Part model, mm, in its own coordinate system. A direction names the side the tool comes from. Coordinates: 2 decimals unless noted, no trailing zeros. Loops run counter-clockwise (first coordinate to the right, second up) from the corner with the lowest first, then second, coordinate; pieces in that order, holes last. Notation, with made-up numbers: (45, -21.5) - (50, -21.5) arc R22 ccw to (50, -4.5) - close; hole circle Ø8 at (56.5, 19). An arc over 180 degrees is marked (long way). Use a Markdown table: item, result. Add a question column.
1. Band-saw the part on A-A, the plane x = 0. Give the cut face in (y, z) (1 decimal), plus the area to 3 significant figures.
2. Drop flat-ended pins along their axis: pin 1 (2.5 mm diameter, centred on y = 15, z = -7.5, fed in from +X); pin 2 (3 mm diameter, centred on x = 9.5, y = 15, fed in from +Z); pin 3 (1.6 mm diameter, centred on y = 16, z = -7, fed in from -X). Give the stop position or say it passes through.
3. Band-saw the part on C-C, the plane y = 32.5. Give the cut face in (x, z) (1 decimal).
4. Wall check: probe 1 along Y at (x, z) = (-9.5, -7.1) (3 decimals); probe 2 along X at (y, z) = (32, 0); probe 3 along X at (y, z) = (6.3, -7.15). Give the ranges that are in metal, low to high. Write a range as [from, to].
5. 3-axis set-ups, long thin cutter, end or side, ignore diameter. For faces 4 (the flat face through (-10, 28.575, -7)), 5 (the flat face through (-8, 19, -5.397)), 6 (the flat face through (0, 9.525, -3)): which of +Z, -Z, +X, -X, +Y, -Y reach the whole face in a straight line?
6. Band-saw the part on D-D, the plane z = 4.5. Give the cut face in (x, y) (3 decimals), plus the area to 3 significant figures.
7. Pull direction Y, two halves, no side cores. Call faces 1 (the cylindrical face through (-11.976, 0.764, -7.007)), 2 (the cylindrical face through (11.516, 30.254, -7.007)), 3 (the flat face through (8, 19, -5.397)): pulls with the +Y half, pulls with the -Y half, needs draft (parallel to the pull), parting line crosses it, or undercut.
8. Band-saw the part on B-B, the plane z = 0. Give the cut face in (x, y) (1 decimal).
from build123d import *

# Parameters (mm, degrees)
SKETCH1_R           = 2.2225
BOSS_EXTRUDE1_DEPTH = 38.1
SKETCH3_W           = 12.7
SKETCH3_H           = 19.05
CUT_EXTRUDE2_DEPTH  = 43.521276806
SKETCH8_W           = 3.81
SKETCH8_H           = 19.05
CUT_EXTRUDE4_DEPTH  = 42.586422571
FILLET1_R           = 2.54
FILLET2_R           = 2.54
FILLET3_R           = 2.54
FILLET4_R           = 2.54
FILLET5_R           = 2.54
FILLET6_R           = 2.54
FILLET7_R           = 2.54
FILLET8_R           = 2.54
SKETCH9_R           = 2.54
CUT_EXTRUDE5_DEPTH  = 43.521276806


with BuildPart() as part:
    # Sketch1 → Boss-Extrude1 (new body)
    with BuildSketch(Plane(origin=(0, 0, 0), x_dir=(1, 0, 0), z_dir=(0, 1, 0))):
        with BuildLine():
            Line((-12.7, 8.572431324), (12.7, 8.572431324))
            Line((12.7, 8.572431324), (12.7, 5.397431324))
            Line((12.7, 5.397431324), (6.600302959, 5.397431324))
            ThreePointArc((6.600302959, 5.397431324), (4.87882252, 4.432224955), (4.804297319, 2.460027138))
            ThreePointArc((4.804297319, 2.460027138), (0, -5.3975), (-4.804297319, 2.460027138))
            ThreePointArc((-4.804297319, 2.460027138), (-4.87882252, 4.432224955), (-6.600302959, 5.397431324))
            Line((-6.600302959, 5.397431324), (-12.7, 5.397431324))
            Line((-12.7, 5.397431324), (-12.7, 8.572431324))
        make_face()
        with Locations(Location((0, 0, 0), (0, 0, 90))):
            Circle(SKETCH1_R, mode=Mode.SUBTRACT)
    extrude(amount=BOSS_EXTRUDE1_DEPTH)

    # Sketch3 → Cut-Extrude2 (cut, through all)
    with BuildSketch(Plane(origin=(0, 0, -8.572431324), x_dir=(-1, 0, 0), z_dir=(0, 0, -1))):
        with Locations((0, 19.05)):
            Rectangle(SKETCH3_W, SKETCH3_H)
    extrude(amount=-CUT_EXTRUDE2_DEPTH, mode=Mode.SUBTRACT)

    # Sketch8 → Cut-Extrude4 (cut, through all)
    with BuildSketch(Plane.XY.offset(-5.397431324)):
        with Locations((-10.795, 19.05)):
            Rectangle(SKETCH8_W, SKETCH8_H)
        with Locations((10.795, 19.05)):
            Rectangle(SKETCH8_W, SKETCH8_H)
    extrude(amount=-CUT_EXTRUDE4_DEPTH, mode=Mode.SUBTRACT)

    # Fillet1
    fillet1_edges = [part.edges().sort_by_distance(p)[0] for p in [
        (12.7, 38.1, -6.984931324),
    ]]
    fillet(fillet1_edges, radius=FILLET1_R)

    # Fillet2
    fillet2_edges = [part.edges().sort_by_distance(p)[0] for p in [
        (-12.7, 38.1, -6.984931324),
    ]]
    fillet(fillet2_edges, radius=FILLET2_R)

    # Fillet3
    fillet3_edges = [part.edges().sort_by_distance(p)[0] for p in [
        (-12.7, 28.575, -6.984931324),
    ]]
    fillet(fillet3_edges, radius=FILLET3_R)

    # Fillet4
    fillet4_edges = [part.edges().sort_by_distance(p)[0] for p in [
        (12.7, 9.525, -6.984931324),
    ]]
    fillet(fillet4_edges, radius=FILLET4_R)

    # Fillet5
    fillet5_edges = [part.edges().sort_by_distance(p)[0] for p in [
        (12.7, 28.575, -6.984931324),
    ]]
    fillet(fillet5_edges, radius=FILLET5_R)

    # Fillet6
    fillet6_edges = [part.edges().sort_by_distance(p)[0] for p in [
        (-12.7, 9.525, -6.984931324),
    ]]
    fillet(fillet6_edges, radius=FILLET6_R)

    # Fillet7
    fillet7_edges = [part.edges().sort_by_distance(p)[0] for p in [
        (-12.7, 0, -6.984931324),
    ]]
    fillet(fillet7_edges, radius=FILLET7_R)

    # Fillet8
    fillet8_edges = [part.edges().sort_by_distance(p)[0] for p in [
        (12.7, 0, -6.984931324),
    ]]
    fillet(fillet8_edges, radius=FILLET8_R)

    # Sketch9 → Cut-Extrude5 (cut, through all)
    with BuildSketch(Plane(origin=(0, 0, -8.572431324), x_dir=(-1, 0, 0), z_dir=(0, 0, -1))):
        with Locations((9.499999999, 31.800000027)):
            Circle(SKETCH9_R)
        with Locations((-9.499999999, 31.800000027)):
            Circle(SKETCH9_R)
        with Locations((9.499999999, 6.299999973)):
            Circle(SKETCH9_R)
        with Locations((-9.499999999, 6.299999973)):
            Circle(SKETCH9_R)
    extrude(amount=-CUT_EXTRUDE5_DEPTH, mode=Mode.SUBTRACT)


solid = part.part
Geometry check:
| question | item | result |
|---|---|---|
| 1 | outline | (0, -8.6) - (9.5, -8.6) - (9.5, -2.2) - (0, -2.2) - close; (0, 2.2) - (9.5, 2.2) - (9.5, 5.4) - (0, 5.4) - close; (28.6, -8.6) - (38.1, -8.6) - (38.1, -2.2) - (28.6, -2.2) - close; (28.6, 2.2) - (38.1, 2.2) - (38.1, 5.4) - (28.6, 5.4) - close |
| 1 | area | 181 mm^2 |
| 2 | pin 1 | stops at x = 8.89 |
| 2 | pin 2 | stops at z = -5.4 |
| 2 | pin 3 | stops at x = -8.89 |
| 3 | outline | (-12.7, -8.6) - (-11.9, -8.6) - (-11.9, -5.4) - (-12.7, -5.4) - close; (-7.1, -8.6) - (7.1, -8.6) - (7.1, -5.4) - (6.6, -5.4) arc R2 cw to (4.8, -2.5) arc R5.4 ccw (long way) to (-4.8, -2.5) arc R2 cw to (-6.6, -5.4) - (-7.1, -5.4) - close; (11.9, -8.6) - (12.7, -8.6) - (12.7, -5.4) - (11.9, -5.4) - close; hole circle Ø4.4 at (0, 0) |
| 4 | probe 1 | y = [0, 3.76], [8.84, 9.525], [28.575, 29.26], [34.34, 38.1] |
| 4 | probe 2 | x = [-5.4, -2.22], [2.22, 5.4] |
| 4 | probe 3 | x = [-12.7, -12.04], [-6.96, 6.96], [12.04, 12.7] |
| 5 | face 4 | +Z, -Z, -X |
| 5 | face 5 | +Z, -X, +Y, -Y |
| 5 | face 6 | +Z, -Z |
| 6 | outline | (-2.98, 0) - (2.98, 0) - (2.98, 9.525) - (-2.98, 9.525) - close; (-2.98, 28.575) - (2.98, 28.575) - (2.98, 38.1) - (-2.98, 38.1) - close |
| 6 | area | 114 mm^2 |
| 7 | face 1 | pulls with the -Y half |
| 7 | face 2 | undercut |
| 7 | face 3 | needs draft |
| 8 | outline | (-5.4, 0) - (-2.2, 0) - (-2.2, 9.5) - (-5.4, 9.5) - close; (-5.4, 28.6) - (-2.2, 28.6) - (-2.2, 38.1) - (-5.4, 38.1) - close; (2.2, 0) - (5.4, 0) - (5.4, 9.5) - (2.2, 9.5) - close; (2.2, 28.6) - (5.4, 28.6) - (5.4, 38.1) - (2.2, 38.1) - close |
